Part model, mm, in its own coordinate system. Face numbers are marked on the shaded views. A direction names the side the tool comes from. Round coordinates to 2 decimals unless told otherwise and drop trailing zeros. Write each loop counter-clockwise with the first axis right and the second up, starting at its lowest first coordinate (ties: lowest second). Pieces come first, ordered by that corner, then holes.
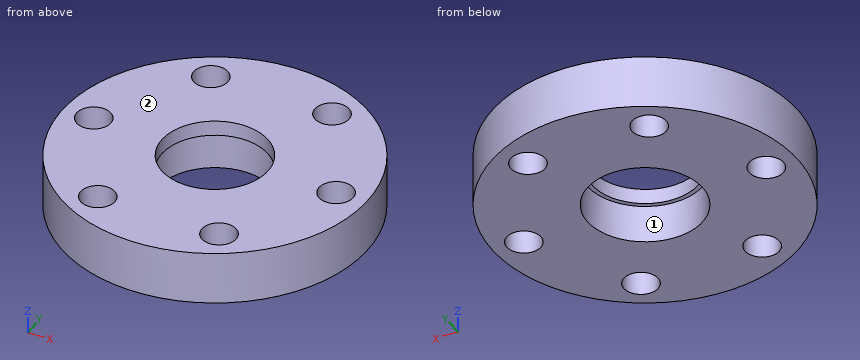
from build123d import *

# Parameters (mm, degrees)
SKETCH1_R           = 20.0025
SKETCH1_R_2         = 7.55
BOSS_EXTRUDE1_DEPTH = 7
SKETCH2_R           = 7.55
SKETCH2_R_2         = 6.952615
BOSS_EXTRUDE2_DEPTH = 2
SKETCH3_R           = 2.25
CUT_EXTRUDE1_DEPTH  = 7


with BuildPart() as part:
    # Sketch1 → Boss-Extrude1 (new body)
    with BuildSketch(Plane(origin=(0, 0, -43.4), x_dir=(-1, 0, 0), z_dir=(0, 0, -1))):
        with Locations(Location((0, 0, 0), (0, 0, 180))):
            Circle(SKETCH1_R)
        with Locations(Location((0, 0, 0), (0, 0, 180))):
            Circle(SKETCH1_R_2, mode=Mode.SUBTRACT)
    extrude(amount=BOSS_EXTRUDE1_DEPTH)

    # Sketch2 → Boss-Extrude2 (add)
    with BuildSketch(Plane(origin=(0, 0, -43.4), x_dir=(-1, 0, 0), z_dir=(0, 0, -1))):
        with Locations(Location((0, 0, 0), (0, 0, 180))):
            Circle(SKETCH2_R)
        Circle(SKETCH2_R_2, mode=Mode.SUBTRACT)
    extrude(amount=BOSS_EXTRUDE2_DEPTH)

    # Sketch3 → Cut-Extrude1 (cut)
    with BuildSketch(Plane(origin=(0, 0, -50.4), x_dir=(-1, 0, 0), z_dir=(0, 0, -1))):
        with Locations((16, 0)):
            Circle(SKETCH3_R)
        with Locations((8, -13.856406461)):
            Circle(SKETCH3_R)
        with Locations((-8, -13.856406461)):
            Circle(SKETCH3_R)
        with Locations((-16, 0)):
            Circle(SKETCH3_R)
        with Locations((-8, 13.856406461)):
            Circle(SKETCH3_R)
        with Locations((8, 13.856406461)):
            Circle(SKETCH3_R)
    extrude(amount=-CUT_EXTRUDE1_DEPTH, mode=Mode.SUBTRACT)


solid = part.part
Q1. Saw through at B-B, the plane y = 4. Write the cut outline in (x, z), and give its area (3 significant figures).
Q2. Saw through at C-C, the plane z = -47.25. Give the number of separate pieces and of enclosed holes in the cut face, and give its area (3 significant figures).
Q3. Drop flat-ended pins along their axis: P1, Ø3, axis at x = -1.5, z = -44.5, coming from the +Y side; P2, Ø1, axis at y = -7, z = -46.5, coming from the -X side; P3, Ø6, axis at x = 8, y = -13.86, coming from the -Z side; P4, Ø1.5, axis at y = 14.5, z = -49.5, coming from the +X side. Give the stop position or say it passes through.
Q4. Saw through at A-A, the plane x = 0. Write the cut outline in (y, z), and give its area (3 significant figures).
Q5. Wall check: line 1 (Y direction, x = 0, z = -48); line 2 (Y direction, x = 8.5, z = -46.25); line 3 (Y direction, x = 8, z = -47.75). Give the ranges that are in metal, low to high.
Q6. Tool access for the marked faces 1 and 2: list every direction of +Z, -Z, +X, -X, +Y, -Y with a clear straight run to the whole face (end or side of a thin tool).
Q7. Saw through at D-D, the plane x = -16. Write the cut outline in (y, z), and give its area (3 significant figures).
Computed:
1. outline: (-19.6, -50.4) - (-6.4, -50.4) - (-6.4, -45.4) - (-5.69, -45.4) - (-5.69, -43.4) - (-19.6, -43.4) - close; (5.69, -45.4) - (6.4, -45.4) - (6.4, -50.4) - (19.6, -50.4) - (19.6, -43.4) - (5.69, -43.4) - close
1. area: 188 mm2
2. separate pieces: 1
2. enclosed holes: 7
2. area: 982 mm2
3. P1: stops at y = 20
3. P2: stops at x = -18.92
3. P3: stops at z = -50.4
3. P4: stops at x = 14.53
4. outline: (-20, -50.4) - (-7.55, -50.4) - (-7.55, -45.4) - (-6.95, -45.4) - (-6.95, -43.4) - (-20, -43.4) - close; (6.95, -45.4) - (7.55, -45.4) - (7.55, -50.4) - (20, -50.4) - (20, -43.4) - (6.95, -43.4) - close
4. area: 177 mm2
5. line 1: y = -20 to -7.55, 7.55 to 20
5. line 2: y = -18.11 to -16.05, -11.66 to 11.66, 16.05 to 18.11
5. line 3: y = -18.33 to -16.11, -11.61 to 11.61, 16.11 to 18.33
6. face 1: -Z
6. face 2: +Z, +X, -X, +Y, -Y
7. outline: (-12, -50.4) - (-2.25, -50.4) - (-2.25, -43.4) - (-12, -43.4) - close; (2.25, -50.4) - (12, -50.4) - (12, -43.4) - (2.25, -43.4) - close
7. area: 137 mm2
